from build123d import *

# Parameters (mm, degrees)
F0_W     = 65
F0_H     = 80
F1_DEPTH = 30
F2_R     = 6.7948556495
F3_DEPTH = 65
F4_R     = 6
F6_T     = -2


# Not quite as in the source:
# - a fillet or chamfer that OpenCascade refuses, or shapes differently, is made with other operations: its cross-section is extruded or revolved along the edge and cut away or added
# - a shell that OpenCascade refuses in one call is made with other operations: the cavity is built on its own and cut out


with BuildPart() as f1:
    # F0 (on Front) → F1 (new body)
    with BuildSketch(Plane.XZ):
        with Locations((32.5, 40)):
            Rectangle(F0_W, F0_H)
    extrude(amount=-F1_DEPTH)

    # F2 (on Right) → F3 (cut, through all)
    with BuildSketch(Plane.YZ):
        with Locations((14.7847002372, 17.048144713)):
            Circle(F2_R)
    extrude(amount=F3_DEPTH, mode=Mode.SUBTRACT)

    # F4
    f4_edges = [f1.edges().sort_by_distance(p)[0] for p in [
        (65, 15, 80),
        (32.5, 0, 80),
        (65, 0, 40),
        (32.5, 0, 0),
        (0, 0, 40),
        (0, 15, 0),
        (0, 30, 40),
        (32.5, 30, 0),
        (65, 15, 0),
        (0, 15, 80),
        (65, 30, 40),
        (32.5, 30, 80),
    ]]
    fillet(f4_edges, radius=F4_R)

    # F5: chamfer of 3 x 6 on 3 edges, made by hand

    # F5_s1 → F5_t2 (revolve, cut)
    with BuildSketch(Plane.XY.offset(17.048144713)):
        Polygon((65, 24.5795558867), (59, 21.5795558867), (65, 21.5795558867), align=None)
    revolve(axis=Axis((65, 14.7847002372, 17.048144713), (1, 0, 0)), mode=Mode.SUBTRACT)

    # F5_s3 → F5_t4 (revolve, cut)
    with BuildSketch(Plane.XY.offset(17.048144713)):
        Polygon((6, 21.5795558867), (0, 24.5795558867), (0, 21.5795558867), align=None)
    revolve(axis=Axis((0, 14.7847002372, 17.048144713), (1, 0, 0)), mode=Mode.SUBTRACT)

    # F6: a shell. OpenCascade refuses it in one call, so the cavity is built on its own and cut out:
    # the body offset inwards by the wall thickness, plus a prism from it out through each open face.
    f6_core = offset(f1.part, amount=F6_T, mode=Mode.PRIVATE)
    f6_exits = [f6_core.faces().sort_by_distance(p)[0] for p in [
        (32.5, 28, 40),
    ]]
    add(f6_core, mode=Mode.SUBTRACT)
    extrude(f6_exits, amount=-F6_T, mode=Mode.SUBTRACT)


solid = f1.part
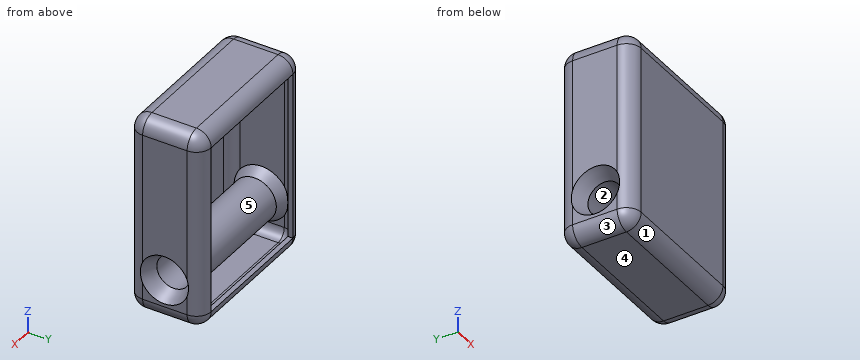
Input: part model. Units: mm. Frame: model coordinates. Face numbers are marked on the shaded views. A direction names the side the tool comes from. Give positions to 0.01 mm unless a question says otherwise; leave off trailing zeros. Order: outer loops, then holes, each group sorted by start corner. A loop starts at its lowest first (then second) coordinate and runs counter-clockwise, first axis right, second up. Notation, with made-up numbers: M 23,5 L 51,5 A19 ccw 51,14 Z; hole C 21,53 d3. An arc over 180 degrees is marked long. Answer as a JSON object with one key per item and string values.
1. Pull-direction query (Y, two-part tool) for the marked faces 1, 2 and 3; classes: +Y half, -Y half, draft (parallel to the pull), parting line (faces both ways), or undercut.
Result sheet:
{"face 1": "-Y half", "face 2": "undercut", "face 3": "draft"}
2. First-contact query: P1, Ø1.5, axis at y = 15.5, z = 9, coming from the -X side; P2, Ø1, axis at y = 29, z = 46.5, coming from the -X side; P3, Ø1.6, axis at y = 28.5, z = 49, coming from the +X side. Flat tips, straight axial feed; report the tip coordinate or a pass-through.
Result sheet:
{"P1": "x = 1.93", "P2": "x = 2.03", "P3": "x = 63.72"}
3. Cut plane B-B, the plane z = 15.5. State how many separate pieces and enclosed holes the cut face has, and give its area (3 significant figures).
Result sheet:
{"separate pieces": "2", "enclosed holes": "1", "area": "419 mm²"}
4. Cut plane A-A, the plane x = 37.5. Output: boundary loops of the cut face in (y, z), and give its area (3 significant figures).
Result sheet:
{"outline": "M 0,6 A6 ccw 6,0 L 24,0 A6 ccw 30,6 L 28,6 A4 cw 24,2 L 6,2 A4 cw 2,6 L 2,74 A4 cw 6,78 L 24,78 A4 cw 28,74 L 30,74 A6 ccw 24,80 L 6,80 A6 ccw 0,74 Z; C 14.78,17.05 d17.59; hole C 14.78,17.05 d13.59", "area": "369 mm²"}
5. Reachability of the marked faces 4 and 5 from +Z, -Z, +X, -X, +Y, -Y: full face, straight path, thin tool, end or side. Return the list, or none.
Result sheet:
{"face 4": "-Z, +X, -X, +Y, -Y", "face 5": "none"}
6. Ray query, line 1 (Y direction, x = 44.5, z = 17); line 2 (Y direction, x = 17, z = 20); line 3 (Z direction, x = 11.5, y = 18). Return the intervals inside material, ascending. Write a range as [from, to].
Result sheet:
{"line 1": "[0, 2], [5.99, 7.99], [21.58, 23.58]", "line 2": "[0, 2], [6.5, 8.66], [20.9, 23.07]", "line 3": "[0, 2], [8.86, 11.06], [23.03, 25.23], [78, 80]"}
7. Cut plane C-C, the plane z = 71. Output: boundary loops of the cut face in (x, y).
Result sheet:
{"outline": "M 0,6 A6 ccw 6,0 L 59,0 A6 ccw 65,6 L 65,24 A6 ccw 59,30 L 59,28 A4 cw 63,24 L 63,6 A4 cw 59,2 L 6,2 A4 cw 2,6 L 2,24 A4 cw 6,28 L 6,30 A6 ccw 0,24 Z"}
